Build history of the part. All positions in model axes, mm. Face numbers are marked on the shaded views. A direction names the side the tool comes from. Coordinates: 2 decimals unless noted, no trailing zeros. Loops run counter-clockwise (first coordinate to the right, second up) from the corner with the lowest first, then second, coordinate; pieces in that order, holes last.
(1) Slice it at B-B (y = -44.45). Give the cut face in (x, z) (3 decimals).
(2) Slice it at C-C (y = -8). Give the cut face in (x, z), and give its area (3 significant figures).
(3) Wall check: L1, parallel to Y at x = -13, z = 332.74 (3 decimals); L2, parallel to Z at x = -8.25, y = -44.45 (3 decimals); L3, parallel to X at y = -40.5, z = 19.5. Give the ranges that are in metal, low to high.
(4) Slice it at A-A (z = 332.74). Give the cut face in (x, y) (3 decimals), and give its area (3 significant figures).
(5) Slice it at D-D (x = -123). Give the cut face in (y, z), and give its area (3 significant figures).
(6) Flat gauge pin, fed straight in: P1, Ø5, axis at x = -93.5, y = -58.5, coming from the +Z side. Where does the tip first touch, or does it go through?
(7) Tool access for the marked faces 1 and 2: list every direction of +Z, -Z, +X, -X, +Y, -Y with a clear straight run to the whole face (end or side of a thin tool).
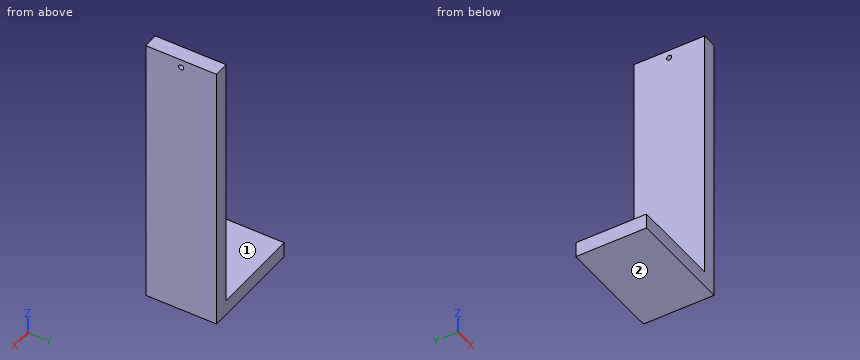
from build123d import *

# Parameters (mm, degrees)
F1_DEPTH = 88.9
F3_D     = 6.35


with BuildPart() as f1:
    # F0 (on Front) → F1 (new body)
    with BuildSketch(Plane.XZ):
        Polygon((-133.35, 0), (0, 0), (0, 342.9), (-19.05, 342.9), (-19.05, 19.05), (-133.35, 19.05), align=None)
    extrude(amount=F1_DEPTH)

    # F3 (through all)
    with Locations(Plane(origin=(-19.05, 0, 0), x_dir=(0, -1, 0), z_dir=(-1, 0, 0))):
        with Locations((44.45, 332.74)):
            Hole(F3_D / 2)


solid = f1.part
Response values:
1. outline: (-133.35, 0) - (0, 0) - (0, 329.565) - (-19.05, 329.565) - (-19.05, 19.05) - (-133.35, 19.05) - close; (-19.05, 335.915) - (0, 335.915) - (0, 342.9) - (-19.05, 342.9) - close
2. outline: (-133.35, 0) - (0, 0) - (0, 342.9) - (-19.05, 342.9) - (-19.05, 19.05) - (-133.35, 19.05) - close
2. area: 8,710 mm2
3. L1: y = -88.9 to -47.625, -41.275 to 0
3. L2: z = 0 to 329.565, 335.915 to 342.9
3. L3: x = -19.05 to 0
4. outline: (-19.05, -88.9) - (0, -88.9) - (0, -47.625) - (-19.05, -47.625) - close; (-19.05, -41.275) - (0, -41.275) - (0, 0) - (-19.05, 0) - close
4. area: 1,570 mm2
5. outline: (-88.9, 0) - (0, 0) - (0, 19.05) - (-88.9, 19.05) - close
5. area: 1,690 mm2
6. P1: stops at z = 19.05
7. face 1: +Z, -X, +Y, -Y
7. face 2: -Z, +X, -X, +Y, -Y
